The listing builds one solid part. Answer for the finished solid, in the listing's coordinates (mm). Coordinates: 2 decimals unless noted, no trailing zeros. Order: outer loops, then holes, each group sorted by start corner. A loop starts at its lowest first (then second) coordinate and runs counter-clockwise, first axis right, second up. Notation, with made-up numbers: (-3, 76) - (33, 76) arc R20 cw to (33, 96) - close; hole circle Ø4 at (-7.75, 40). An arc over 180 degrees is marked (long way). Use a Markdown table: item, result. Add a question column.
Item 1: Find the intervals of material crossed by line 1 along X through (y, z) = (2.45, 25.5); line 2 along X through (y, z) = (1.1, 18.5); line 3 along Z through (x, y) = (-72, 0.7), in increasing order.
Item 2: The part is cut by section C-C, the plane z = 7. Give the vertices of the cut face in (x, y).
Item 3: The part is cut by section D-D, the plane y = 2.1. State how many separate pieces and enclosed holes the cut face has, then the cut area to 3 significant figures.
Item 4: The mould has two halves that part along Z. Classify faces 1 (the flat face through (76.57, 1.52, -13.49)), 2 (the cylindrical face through (-41.6, 1.52, -13.72)), 3 (the flat face through (-1, 0, 0)), 4 (the cylindrical face through (4.35, 1.52, 27.07)): released by +Z, released by -Z, zero draft, split by the parting line, or undercut.
Item 5: Flat-ended cylindrical pins translate along their axes: P1, Ø1.5, axis at x = -97, y = 1, coming from the -Z side; P2, Ø1.5, axis at y = 1, z = -29.5, coming from the -X side; P3, Ø1, axis at x = -57.5, y = 0.5, coming from the -Z side. Find the tip coordinate at first contact, or state that the pin passes through.
Item 6: The part is cut by section B-B, the plane z = 25.5. Give the vertices of the cut face in (x, y), then the cut area to 3 significant figures.
Item 7: The part is cut by section A-A, the plane x = -40.09. Give the vertices of the cut face in (y, z), then the cut area to 3 significant figures.
from build123d import *

# Parameters (mm, degrees)
SKETCH1_W           = 196
SKETCH1_H           = 61
BOSS_EXTRUDE1_DEPTH = 3
SKETCH2_R           = 1.7
SKETCH2_W           = 30
SKETCH2_H           = 47.5
SKETCH2_W_2         = 3
SKETCH2_H_2         = 10
SKETCH2_H_3         = 11
SKETCH2_H_4         = 3
CUT_EXTRUDE1_DEPTH  = 3
CUT_EXTRUDE2_DEPTH  = 10
BOSS_EXTRUDE2_DEPTH = 3


with BuildPart() as part:
    # Sketch1 → Boss-Extrude1 (new body)
    with BuildSketch(Plane(origin=(0, 0, 0), x_dir=(1, 0, 0), z_dir=(0, 1, 0))):
        Rectangle(SKETCH1_W, SKETCH1_H)
    extrude(amount=BOSS_EXTRUDE1_DEPTH)

    # Sketch2 → Cut-Extrude1 (cut)
    with BuildSketch(Plane(origin=(0, 3, 0), x_dir=(1, 0, 0), z_dir=(0, 1, 0))):
        with Locations(Location((-40.09, 14.5, 0), (0, 0, 270))):
            Circle(SKETCH2_R)
        with Locations(Location((5, -25.5, 0), (0, 0, 270))):
            Circle(SKETCH2_R)
        with Locations((-64.4, -6.75)):
            Rectangle(SKETCH2_W, SKETCH2_H)
        with Locations((-96.5, 25.5)):
            Rectangle(SKETCH2_W_2, SKETCH2_H_2)
        with Locations((-96.5, 0.5)):
            Rectangle(SKETCH2_W_2, SKETCH2_H_2)
        with Locations((-96.5, -25)):
            Rectangle(SKETCH2_W_2, SKETCH2_H_3)
        with Locations((96.5, 0.5)):
            Rectangle(SKETCH2_W_2, SKETCH2_H_2)
        with Locations((96.5, -25)):
            Rectangle(SKETCH2_W_2, SKETCH2_H_3)
        with Locations((-3, 29)):
            Rectangle(SKETCH2_W, SKETCH2_H_4)
        with Locations((-63, 29)):
            Rectangle(SKETCH2_W, SKETCH2_H_4)
        with Locations((57, 29)):
            Rectangle(SKETCH2_W, SKETCH2_H_4)
        with Locations((96.5, 25.5)):
            Rectangle(SKETCH2_W_2, SKETCH2_H_2)
    extrude(amount=-CUT_EXTRUDE1_DEPTH, mode=Mode.SUBTRACT)

    # Sketch3 → Cut-Extrude2 (cut)
    with BuildSketch(Plane(origin=(0, 3, 0), x_dir=(1, 0, 0), z_dir=(0, 1, 0))):
        Polygon((12, 30.5), (98, 30.5), (98, 5.5), (95, 5.5), (85.333795578, 8.062126473), (86.10243352, 10.9619878), (66.770024675, 16.086240747), (66.001386733, 13.18637942), (40.998613267, 19.81362058), (41.767251209, 22.713481907), (22.434842364, 27.837734853), (21.666204422, 24.937873527), (12, 27.5), align=None)
    extrude(amount=-CUT_EXTRUDE2_DEPTH, mode=Mode.SUBTRACT)

    # Sketch5 → Boss-Extrude2 (add)
    with BuildSketch(Plane(origin=(0, 3, 0), x_dir=(1, 0, 0), z_dir=(0, 1, 0))):
        Polygon((12, 27.5), (0.681818182, 30.5), (0.681818182, 27.5), align=None)
    extrude(amount=-BOSS_EXTRUDE2_DEPTH)


solid = part.part
Solution:
| question | item | result |
|---|---|---|
| 1 | line 1 | x = -95 to -79.4, -49.4 to 3.3, 6.7 to 95 |
| 1 | line 2 | x = -98 to -79.4, -49.4 to 98 |
| 1 | line 3 | z = -27.5 to -17 |
| 2 | outline | (-98, 0) - (-79.4, 0) - (-79.4, 3) - (-98, 3) - close; (-49.4, 0) - (98, 0) - (98, 3) - (-49.4, 3) - close |
| 3 | separate pieces | 1 |
| 3 | enclosed holes | 2 |
| 3 | area | 9,080 mm2 |
| 4 | face 1 | released by -Z |
| 4 | face 2 | undercut |
| 4 | face 3 | zero draft |
| 4 | face 4 | undercut |
| 5 | P1 | stops at z = -20.5 |
| 5 | P2 | stops at x = -95 |
| 5 | P3 | stops at z = -27.5 |
| 6 | outline | (-95, 0) - (-79.4, 0) - (-79.4, 3) - (-95, 3) - close; (-49.4, 0) - (3.3, 0) - (3.3, 3) - (-49.4, 3) - close; (6.7, 0) - (95, 0) - (95, 3) - (6.7, 3) - close |
| 6 | area | 470 mm2 |
| 7 | outline | (0, -30.5) - (3, -30.5) - (3, -16.2) - (0, -16.2) - close; (0, -12.8) - (3, -12.8) - (3, 30.5) - (0, 30.5) - close |
| 7 | area | 173 mm2 |
